```python
from build123d import *

# Parameters (mm, degrees)
EXTRUDE_1_DEPTH          = 3
SKETCH_2_R               = 11
CUT_EXTRUDE_1_DEPTH      = 4
SKETCH_5_R               = 20
SKETCH_5_R_2             = 18
EXTRUDE_2_DEPTH          = 5
PATTERN_CIRCULAR_1_COUNT = 4
CHAMFER_1_SIZE           = 0.5


with BuildPart() as part:
    # Эскиз1 → Бобышка-Вытянуть1 (new body)
    with BuildSketch(Plane.XY):
        with BuildLine():
            ThreePointArc((-17.685483871, -3.350173167), (-12.727922061, -12.727922061), (-3.350173167, -17.685483871))
            ThreePointArc((-3.350173167, -17.685483871), (10.136595409, -14.874455738), (17.685483871, -3.350173167))
            ThreePointArc((17.685483871, -3.350173167), (12.727922061, 12.727922061), (-3.350173167, 17.685483871))
            ThreePointArc((-3.350173167, 17.685483871), (-14.874455738, 10.136595409), (-17.685483871, -3.350173167))
        make_face()
    extrude(amount=EXTRUDE_1_DEPTH)

    # Эскиз2 → Вырез-Вытянуть1 (cut, through all)
    with BuildSketch(Plane.XY.offset(3)):
        Circle(SKETCH_2_R)
    extrude(amount=-CUT_EXTRUDE_1_DEPTH, mode=Mode.SUBTRACT)

    # Эскиз5 → Бобышка-Вытянуть2 (add)
    with BuildSketch(Plane.XY.offset(3)):
        Circle(SKETCH_5_R)
        Circle(SKETCH_5_R_2, mode=Mode.SUBTRACT)
    extrude(amount=-EXTRUDE_2_DEPTH)

    # Эскиз6 → Вырез-Повернуть1 (revolve, cut)
    with BuildSketch(Plane(origin=(0, 0, 0), x_dir=(1, 0, 0), z_dir=(0, 1, 0))):
        Polygon((-16.6, -1.648035715), (-18, -3), (-15.5, -3), (-15.5, -1.648035715), (-15.5, 2), (-16.6, 2), align=None)
    cut_revolve_1 = revolve(axis=Axis((-15.5, 0, -24.0808518), (0, 0, 1)), mode=Mode.SUBTRACT)

    # Круговой массив1: Вырез-Повернуть1 ×4 about axis
    pattern_circular_1_axis = Axis((0, 0, 0), (0, 0, 1))
    for i in range(1, PATTERN_CIRCULAR_1_COUNT):
        add(cut_revolve_1.rotate(pattern_circular_1_axis, i * 360 / PATTERN_CIRCULAR_1_COUNT), mode=Mode.SUBTRACT)

    # Фаска1
    chamfer_1_edges = [part.edges().sort_by_distance(p)[0] for p in [
        (-18, 0, -2),
    ]]
    chamfer(chamfer_1_edges, length=CHAMFER_1_SIZE)


solid = part.part
```
CAD build for the part. Positions are in the model's coordinates, mm. A direction names the side the tool comes from. Round coordinates to 2 decimals unless told otherwise and drop trailing zeros. Write each loop counter-clockwise with the first axis right and the second up, starting at its lowest first coordinate (ties: lowest second). Pieces come first, ordered by that corner, then holes. Notation, with made-up numbers: (17, 11) -> (55, 11) arc R13 ccw to (55, 22) -> close; hole circle Ø5 at (74.25, 29.5). An arc over 180 degrees is marked (long way). Answer in a Markdown table with one row per item. Add a question column.
Item 1: Saw through at B-B, the plane z = 1. Write the cut outline in (x, y).
Item 2: Saw through at A-A, the plane y = 0. Write the cut outline in (x, z), then the cut area to 3 significant figures.
Item 3: Drop flat-ended pins along their axis: pin 1 Ø2 at (x, z) = (-9, -0.5) entering from -Y; pin 2 Ø1.5 at (x, y) = (-13, 11) entering from -Z; pin 3 Ø3.5 at (x, y) = (15.5, 0) entering from +Z. Give the stop position or say it passes through.
Item 4: Drill centre lines: line 1 (Y direction, x = 0, z = -1.05); line 2 (Z direction, x = -3.5, y = -13); line 3 (Y direction, x = -2, z = 2.05). Where is each one in solid material? Low to high. Write a range as from..to.
Item 5: Which spindle directions (+Z, -Z, +X, -X, +Y, -Y) get a long thin tool onto all of the face, cutting with end or side? Do faces 5 (the face through (0, -14.4, 0.8)), 6 (the face through (8, 8, 0)). Say none if no direction does.
Item 6: Mould opens along X. For faces 1 (the face through (0, 14.4, 0.8)), 2 (the face through (-4.336, -19.524, 0.535)), 3 (the face through (9, -9, 3)), 4 (the face through (-2.38, -10.74, 1.52)) say: pulls with the +X half, pulls with the -X half, needs draft (parallel to the pull), parting line crosses it, or undercut.
Findings below:
| question | item | result |
|---|---|---|
| 1 | outline | circle Ø40 at (0, 0); hole circle Ø2.2 at (-15.5, 0); hole circle Ø22 at (0, 0); hole circle Ø2.2 at (0, -15.5); hole circle Ø2.2 at (0, 15.5); hole circle Ø2.2 at (15.5, 0) |
| 2 | outline | (-20, -2) -> (-18.5, -2) -> (-18, -1.5) -> (-18, 0) -> (-16.6, 0) -> (-16.6, 1.65) -> (-18, 3) -> (-20, 3) -> close; (-14.4, 0) -> (-11, 0) -> (-11, 3) -> (-13, 3) -> (-14.4, 1.65) -> close; (11, 0) -> (14.4, 0) -> (14.4, 1.65) -> (13, 3) -> (11, 3) -> close; (16.6, 0) -> (18, 0) -> (18, -1.5) -> (18.5, -2) -> (20, -2) -> (20, 3) -> (18, 3) -> (16.6, 1.65) -> close |
| 2 | area | 44.8 mm^2 |
| 3 | pin 1 | stops at y = -18.33 |
| 3 | pin 2 | stops at z = 0 |
| 3 | pin 3 | stops at z = 2.28 |
| 4 | line 1 | y = -20..-18, 18..20 |
| 4 | line 2 | z = 0..3 |
| 4 | line 3 | y = -19.9..-10.82, 10.82..19.9 |
| 5 | face 5 | +Z, -Z |
| 5 | face 6 | -Z |
| 6 | face 1 | undercut |
| 6 | face 2 | parting line crosses it |
| 6 | face 3 | needs draft |
| 6 | face 4 | undercut |
